```python
from build123d import *

# Parameters (mm, degrees)
SKETCH_W        = 980
SKETCH_H        = 480
PAD_DEPTH       = 1
SKETCH077_R     = 1.9
SKETCH077_W     = 103.6
SKETCH077_H     = 177.6
POCKET018_DEPTH = 1
SKETCH095_R     = 1.9
SKETCH095_W     = 103.6
SKETCH095_H     = 177.6
POCKET023_DEPTH = 1
SKETCH113_R     = 1.9
SKETCH113_W     = 103.6
SKETCH113_H     = 177.6
POCKET028_DEPTH = 1
SKETCH131_R     = 1.9
SKETCH131_W     = 103.6
SKETCH131_H     = 177.6
POCKET033_DEPTH = 1
SKETCH149_R     = 1.9
SKETCH149_W     = 103.6
SKETCH149_H     = 177.6
POCKET038_DEPTH = 1
SKETCH198_R     = 1.9
SKETCH198_W     = 57.6
SKETCH198_H     = 107.6
POCKET056_DEPTH = 1
SKETCH216_R     = 1.9
SKETCH216_W     = 103.6
SKETCH216_H     = 177.6
POCKET061_DEPTH = 1
SKETCH234_R     = 1.9
SKETCH234_W     = 103.6
SKETCH234_H     = 177.6
POCKET066_DEPTH = 1
SKETCH252_R     = 1.9
SKETCH252_W     = 103.6
SKETCH252_H     = 177.6
POCKET071_DEPTH = 1
SKETCH270_R     = 1.9
SKETCH270_W     = 103.6
SKETCH270_H     = 177.6
POCKET076_DEPTH = 1
SKETCH288_R     = 1.9
SKETCH288_W     = 103.6
SKETCH288_H     = 177.6
POCKET081_DEPTH = 1
SKETCH303_R     = 1.9
SKETCH303_W     = 57.6
SKETCH303_H     = 107.6
POCKET085_DEPTH = 1


with BuildPart() as part:
    # Sketch → Pad (new body)
    with BuildSketch(Plane.XY):
        Rectangle(SKETCH_W, SKETCH_H)
    extrude(amount=PAD_DEPTH)

    # Sketch077 (on Face5 of Pad) → Pocket018 (cut)
    with BuildSketch(Plane(origin=(0, 0, 0), x_dir=(1, 0, 0), z_dir=(0, 0, -1))):
        with Locations((459.999969, -41.999985)):
            Circle(SKETCH077_R)
        with Locations((459.999969, -119.999985)):
            Circle(SKETCH077_R)
        with Locations((459.999969, -197.999985)):
            Circle(SKETCH077_R)
        with Locations((333.999969, -167.999985)):
            Circle(SKETCH077_R)
        with Locations((333.999969, -71.999985)):
            Circle(SKETCH077_R)
        with Locations((396.999969, -119.999985)):
            Rectangle(SKETCH077_W, SKETCH077_H)
    extrude(amount=-POCKET018_DEPTH, mode=Mode.SUBTRACT)

    # Sketch095 (on Face4 of Pocket018) → Pocket023 (cut)
    with BuildSketch(Plane(origin=(0, 0, 0), x_dir=(1, 0, 0), z_dir=(0, 0, -1))):
        with Locations((309.999924, -42.000008)):
            Circle(SKETCH095_R)
        with Locations((309.999924, -120.000008)):
            Circle(SKETCH095_R)
        with Locations((183.999924, -72.000008)):
            Circle(SKETCH095_R)
        with Locations((309.999924, -198.000008)):
            Circle(SKETCH095_R)
        with Locations((183.999924, -168.000008)):
            Circle(SKETCH095_R)
        with Locations((246.999924, -120.000008)):
            Rectangle(SKETCH095_W, SKETCH095_H)
    extrude(amount=-POCKET023_DEPTH, mode=Mode.SUBTRACT)

    # Sketch113 (on Face4 of Pocket023) → Pocket028 (cut)
    with BuildSketch(Plane(origin=(0, 0, 0), x_dir=(1, 0, 0), z_dir=(0, 0, -1))):
        with Locations((159.999886, -120.000023)):
            Circle(SKETCH113_R)
        with Locations((159.999886, -42.000023)):
            Circle(SKETCH113_R)
        with Locations((159.999886, -198.000023)):
            Circle(SKETCH113_R)
        with Locations((33.999886, -168.000023)):
            Circle(SKETCH113_R)
        with Locations((33.999886, -72.000023)):
            Circle(SKETCH113_R)
        with Locations((96.999886, -120.000023)):
            Rectangle(SKETCH113_W, SKETCH113_H)
    extrude(amount=-POCKET028_DEPTH, mode=Mode.SUBTRACT)

    # Sketch131 (on Face4 of Pocket028) → Pocket033 (cut)
    with BuildSketch(Plane(origin=(0, 0, 0), x_dir=(1, 0, 0), z_dir=(0, 0, -1))):
        with Locations((-20.000153, -42.000076)):
            Circle(SKETCH131_R)
        with Locations((-20.000153, -120.000076)):
            Circle(SKETCH131_R)
        with Locations((-20.000153, -198.000076)):
            Circle(SKETCH131_R)
        with Locations((-146.000153, -168.000076)):
            Circle(SKETCH131_R)
        with Locations((-146.000153, -72.000076)):
            Circle(SKETCH131_R)
        with Locations((-83.000153, -120.000076)):
            Rectangle(SKETCH131_W, SKETCH131_H)
    extrude(amount=-POCKET033_DEPTH, mode=Mode.SUBTRACT)

    # Sketch149 (on Face4 of Pocket033) → Pocket038 (cut)
    with BuildSketch(Plane(origin=(0, 0, 0), x_dir=(1, 0, 0), z_dir=(0, 0, -1))):
        with Locations((-150.000107, -42.000069)):
            Circle(SKETCH149_R)
        with Locations((-150.000107, -120.000069)):
            Circle(SKETCH149_R)
        with Locations((-150.000107, -198.000069)):
            Circle(SKETCH149_R)
        with Locations((-276.000107, -168.000069)):
            Circle(SKETCH149_R)
        with Locations((-276.000107, -72.000069)):
            Circle(SKETCH149_R)
        with Locations((-213.000107, -120.000069)):
            Rectangle(SKETCH149_W, SKETCH149_H)
    extrude(amount=-POCKET038_DEPTH, mode=Mode.SUBTRACT)

    # Sketch198 (on Face5 of Pad) → Pocket056 (cut)
    with BuildSketch(Plane(origin=(0, 0, 0), x_dir=(1, 0, 0), z_dir=(0, 0, -1))):
        with Locations((-276.000183, -86.000107)):
            Circle(SKETCH198_R)
        with Locations((-276.000183, -154.000107)):
            Circle(SKETCH198_R)
        with Locations((-356.000183, -66.000107)):
            Circle(SKETCH198_R)
        with Locations((-356.000183, -174.000107)):
            Circle(SKETCH198_R)
        with Locations((-316.000183, -120.000107)):
            Rectangle(SKETCH198_W, SKETCH198_H)
    extrude(amount=-POCKET056_DEPTH, mode=Mode.SUBTRACT)

    # Sketch216 (on Face5 of Pad) → Pocket061 (cut)
    with BuildSketch(Plane(origin=(0, 0, 0), x_dir=(1, 0, 0), z_dir=(0, 0, -1))):
        with Locations((459.999878, 42.000061)):
            Circle(SKETCH216_R)
        with Locations((333.999878, 72.000061)):
            Circle(SKETCH216_R)
        with Locations((333.999878, 168.000061)):
            Circle(SKETCH216_R)
        with Locations((459.999878, 198.000061)):
            Circle(SKETCH216_R)
        with Locations((459.999878, 120.000061)):
            Circle(SKETCH216_R)
        with Locations((396.999878, 120.000061)):
            Rectangle(SKETCH216_W, SKETCH216_H)
    extrude(amount=-POCKET061_DEPTH, mode=Mode.SUBTRACT)

    # Sketch234 (on Face4 of Pocket061) → Pocket066 (cut)
    with BuildSketch(Plane(origin=(0, 0, 0), x_dir=(1, 0, 0), z_dir=(0, 0, -1))):
        with Locations((309.999893, 198.000046)):
            Circle(SKETCH234_R)
        with Locations((183.999893, 168.000046)):
            Circle(SKETCH234_R)
        with Locations((309.999893, 120.000046)):
            Circle(SKETCH234_R)
        with Locations((309.999893, 42.000046)):
            Circle(SKETCH234_R)
        with Locations((183.999893, 72.000046)):
            Circle(SKETCH234_R)
        with Locations((246.999893, 120.000046)):
            Rectangle(SKETCH234_W, SKETCH234_H)
    extrude(amount=-POCKET066_DEPTH, mode=Mode.SUBTRACT)

    # Sketch252 (on Face4 of Pocket066) → Pocket071 (cut)
    with BuildSketch(Plane(origin=(0, 0, 0), x_dir=(1, 0, 0), z_dir=(0, 0, -1))):
        with Locations((159.999924, 198.000069)):
            Circle(SKETCH252_R)
        with Locations((159.999924, 120.000069)):
            Circle(SKETCH252_R)
        with Locations((159.999924, 42.000069)):
            Circle(SKETCH252_R)
        with Locations((33.999924, 72.000069)):
            Circle(SKETCH252_R)
        with Locations((33.999924, 168.000069)):
            Circle(SKETCH252_R)
        with Locations((96.999924, 120.000069)):
            Rectangle(SKETCH252_W, SKETCH252_H)
    extrude(amount=-POCKET071_DEPTH, mode=Mode.SUBTRACT)

    # Sketch270 (on Face4 of Pocket071) → Pocket076 (cut)
    with BuildSketch(Plane(origin=(0, 0, 0), x_dir=(1, 0, 0), z_dir=(0, 0, -1))):
        with Locations((-146.000107, 168)):
            Circle(SKETCH270_R)
        with Locations((-146.000107, 72)):
            Circle(SKETCH270_R)
        with Locations((-20.000107, 42)):
            Circle(SKETCH270_R)
        with Locations((-20.000107, 120)):
            Circle(SKETCH270_R)
        with Locations((-20.000107, 198)):
            Circle(SKETCH270_R)
        with Locations((-83.000107, 120)):
            Rectangle(SKETCH270_W, SKETCH270_H)
    extrude(amount=-POCKET076_DEPTH, mode=Mode.SUBTRACT)

    # Sketch288 (on Face4 of Pocket076) → Pocket081 (cut)
    with BuildSketch(Plane(origin=(0, 0, 0), x_dir=(1, 0, 0), z_dir=(0, 0, -1))):
        with Locations((-150.000107, 197.999969)):
            Circle(SKETCH288_R)
        with Locations((-150.000107, 119.999969)):
            Circle(SKETCH288_R)
        with Locations((-150.000107, 41.999969)):
            Circle(SKETCH288_R)
        with Locations((-276.000107, 71.999969)):
            Circle(SKETCH288_R)
        with Locations((-276.000107, 167.999969)):
            Circle(SKETCH288_R)
        with Locations((-213.000107, 119.999969)):
            Rectangle(SKETCH288_W, SKETCH288_H)
    extrude(amount=-POCKET081_DEPTH, mode=Mode.SUBTRACT)

    # Sketch303 (on Face4 of Pocket081) → Pocket085 (cut)
    with BuildSketch(Plane(origin=(0, 0, 0), x_dir=(1, 0, 0), z_dir=(0, 0, -1))):
        with Locations((-276.000275, 85.999939)):
            Circle(SKETCH303_R)
        with Locations((-356.000275, 65.999939)):
            Circle(SKETCH303_R)
        with Locations((-276.000275, 153.999939)):
            Circle(SKETCH303_R)
        with Locations((-356.000275, 173.999939)):
            Circle(SKETCH303_R)
        with Locations((-316.000275, 119.999939)):
            Rectangle(SKETCH303_W, SKETCH303_H)
    extrude(amount=-POCKET085_DEPTH, mode=Mode.SUBTRACT)


solid = part.part
```
The listing builds one solid part. Answer for the finished solid, in the listing's coordinates (mm). Round coordinates to 2 decimals unless told otherwise and drop trailing zeros. Loops run counter-clockwise (first coordinate to the right, second up) from the corner with the lowest first, then second, coordinate; pieces in that order, holes last. Notation, with made-up numbers: (14.5, 33.25) - (71.5, 33.25) arc R28 ccw to (71.5, 55.25) - close; hole circle Ø11 at (-9, 32). An arc over 180 degrees is marked (long way). Return JSON: item names as keys, results as strings. Group by question number.
1. The part is cut by section C-C on z = 0.5. State how many separate pieces and enclosed holes the cut face has, then the cut area to 3 significant figures.
2. The part is cut by section B-B on y = 104. Determine the outline of the cut face in (x, z), then the cut area to 3 significant figures.
3. The part is cut by section A-A on x = -248. Determine the outline of the cut face in (y, z).
4. Consider probe 1 along X at (y, z) = (182, 0.5); probe 2 along Y at (x, z) = (243.5, 0.2). Determine where each line is inside the solid, lowest interval first.
Resolved:
{
 "1": {"separate pieces": "1", "enclosed holes": "70", "area": "273,000 mm²"},
 "2": {"outline": "(-490, 0) - (-344.8, 0) - (-344.8, 1) - (-490, 1) - close; (-287.2, 0) - (-264.8, 0) - (-264.8, 1) - (-287.2, 1) - close; (-161.2, 0) - (-134.8, 0) - (-134.8, 1) - (-161.2, 1) - close; (-31.2, 0) - (45.2, 0) - (45.2, 1) - (-31.2, 1) - close; (148.8, 0) - (195.2, 0) - (195.2, 1) - (148.8, 1) - close; (298.8, 0) - (345.2, 0) - (345.2, 1) - (298.8, 1) - close; (448.8, 0) - (490, 0) - (490, 1) - (448.8, 1) - close", "area": "404 mm²"},
 "3": {"outline": "(-240, 0) - (-208.8, 0) - (-208.8, 1) - (-240, 1) - close; (-31.2, 0) - (31.2, 0) - (31.2, 1) - (-31.2, 1) - close; (208.8, 0) - (240, 0) - (240, 1) - (208.8, 1) - close"},
 "4": {"probe 1": "x = -490 to -264.8, -161.2 to -134.8, -31.2 to 45.2, 148.8 to 195.2, 298.8 to 345.2, 448.8 to 490", "probe 2": "y = -240 to -208.8, -31.2 to 31.2, 208.8 to 240"}
}
